```python
from build123d import *

# Parameters (mm, degrees)
SKETCH007_R   = 1.7
PAD004_DEPTH  = 2
SKETCH009_W   = 32
SKETCH009_H   = 24
PAD005_DEPTH  = 2
SKETCH010_R   = 0.6
HOLE001_DEPTH = 25


with BuildPart() as part:
    # Sketch007 (on Face8 of ShapeBinder001) → Pad004 (new body)
    with BuildSketch(Plane(origin=(2, -20, 0), x_dir=(0, 0, -1), z_dir=(0, -1, 0))):
        with BuildLine():
            ThreePointArc((5, 9.9), (0.1, 5), (5, 0.1))
            Line((15, 0.1), (5, 0.1))
            Line((15, 9.9), (15, 0.1))
            Line((5, 9.9), (15, 9.9))
        make_face()
        with Locations((5, 5)):
            Circle(SKETCH007_R, mode=Mode.SUBTRACT)
    extrude(amount=PAD004_DEPTH)

    # Sketch009 (on Face4 of Pad004) → Pad005 (join)
    with BuildSketch(Plane(origin=(2, 0, -15), x_dir=(0, 1, 0), z_dir=(0, 0, -1))):
        with Locations((-36, 4.339121)):
            Rectangle(SKETCH009_W, SKETCH009_H)
    extrude(amount=PAD005_DEPTH)

    # Sketch010 (on Face10 of Pad005) → Hole001 (cut)
    with BuildSketch(Plane(origin=(2, 0, -17), x_dir=(0, 1, 0), z_dir=(0, 0, -1))):
        with Locations((-50, 14.339121)):
            Circle(SKETCH010_R)
        with Locations((-22, 14.339121)):
            Circle(SKETCH010_R)
        with Locations((-22, -5.660879)):
            Circle(SKETCH010_R)
        with Locations((-50, -5.660879)):
            Circle(SKETCH010_R)
    extrude(amount=-HOLE001_DEPTH, mode=Mode.SUBTRACT)


solid = part.part
```
Could you check a few things on this model? Use its own coordinates, in mm. A direction names the side the tool comes from. Coordinates: 2 decimals unless noted, no trailing zeros. Loops run counter-clockwise (first coordinate to the right, second up) from the corner with the lowest first, then second, coordinate; pieces in that order, holes last. Notation, with made-up numbers: M -3.75,-12 L 24.25,-12 A33 ccw 24.25,16 Z; hole C 54,30.5 d6. An arc over 180 degrees is marked long. Put each result on its own line as item: value. Start each with the question number.
(1) Will these pins go through, and if not, where does the flat tip stop? P1, Ø8, axis at x = 7, z = -5.5, coming from the -Y side; P2, Ø10, axis at x = 10.5, z = -11, coming from the -Y side; P3, Ø1, axis at y = -21, z = -9.5, coming from the -X side; P4, Ø1.5, axis at x = 8.5, y = -23.5, coming from the +Z side.
(2) For faces 1 (the face through (11.9, -21, -10)), 2 (the face through (2.1, -21, -10)), 3 (the face through (7, -22, -7)), which set-ups out of +Z, -Z, +X, -X, +Y, -Y let a thin tool reach every point of the face, with its end or its side?
(3) Suppose I cut it at B-B on x = 7. Please give me the cut outline in (y, z), then the cut area to 3 significant figures.
(4) Suppose I cut it at C-C on z = -9.5. Please give me the cut outline in (x, y).
(5) Thinking about a two-plate mould opening in Y: for faces 4 (the face through (6, -52, -16)), 5 (the face through (18.339, -36, -16)), 6 (the face through (15.974, -50.476, -16.014)), which applies, pulls with the +Y half, pulls with the -Y half, needs draft (parallel to the pull), parting line crosses it, or undercut?
(6) Suppose I cut it at D-D on y = -35. Please give me the cut outline in (x, z).
(7) I need wall thicknesses on line 1 (X direction, y = -50, z = -16.4); line 2 (X direction, y = -20.85, z = -5); line 3 (Y direction, x = 5, z = -10.75). Which ranges of each line are inside material? Lowest first, please. Write a range as from..to.
(8) Suppose I cut it at A-A on y = -50. Please give me the cut outline in (x, z), then the cut area to 3 significant figures.
Solutions:
1. P1: stops at y = -22
1. P2: stops at y = -52
1. P3: stops at x = 2.1
1. P4: stops at z = -15
2. face 1: +Z, +X, +Y, -Y
2. face 2: +Z, -X, +Y, -Y
2. face 3: +Z, +X, -X, -Y
3. outline: M -52,-17 L -20,-17 L -20,-6.7 L -22,-6.7 L -22,-15 L -52,-15 Z; M -22,-3.3 L -20,-3.3 L -20,-0.1 L -22,-0.1 Z
3. area: 87.0 mm2
4. outline: M 2.1,-22 L 11.9,-22 L 11.9,-20 L 2.1,-20 Z
5. face 4: pulls with the -Y half
5. face 5: needs draft
5. face 6: undercut
6. outline: M -5.66,-17 L 18.34,-17 L 18.34,-15 L -5.66,-15 Z
7. line 1: x = -5.66..-4.26, -3.06..15.74, 16.94..18.34
7. line 2: x = 2.1..5.3, 8.7..11.9
7. line 3: y = -22..-20
8. outline: M -5.66,-17 L -4.26,-17 L -4.26,-15 L -5.66,-15 Z; M -3.06,-17 L 15.74,-17 L 15.74,-15 L -3.06,-15 Z; M 16.94,-17 L 18.34,-17 L 18.34,-15 L 16.94,-15 Z
8. area: 43.2 mm2
